Source: three-view drawing plus pictorial views. Frame: mm from the lowest corner of the part. Give positions to 0.01 mm unless a question says otherwise; leave off trailing zeros. Write each loop counter-clockwise with the first axis right and the second up, starting at its lowest first coordinate (ties: lowest second). Pieces come first, ordered by that corner, then holes.
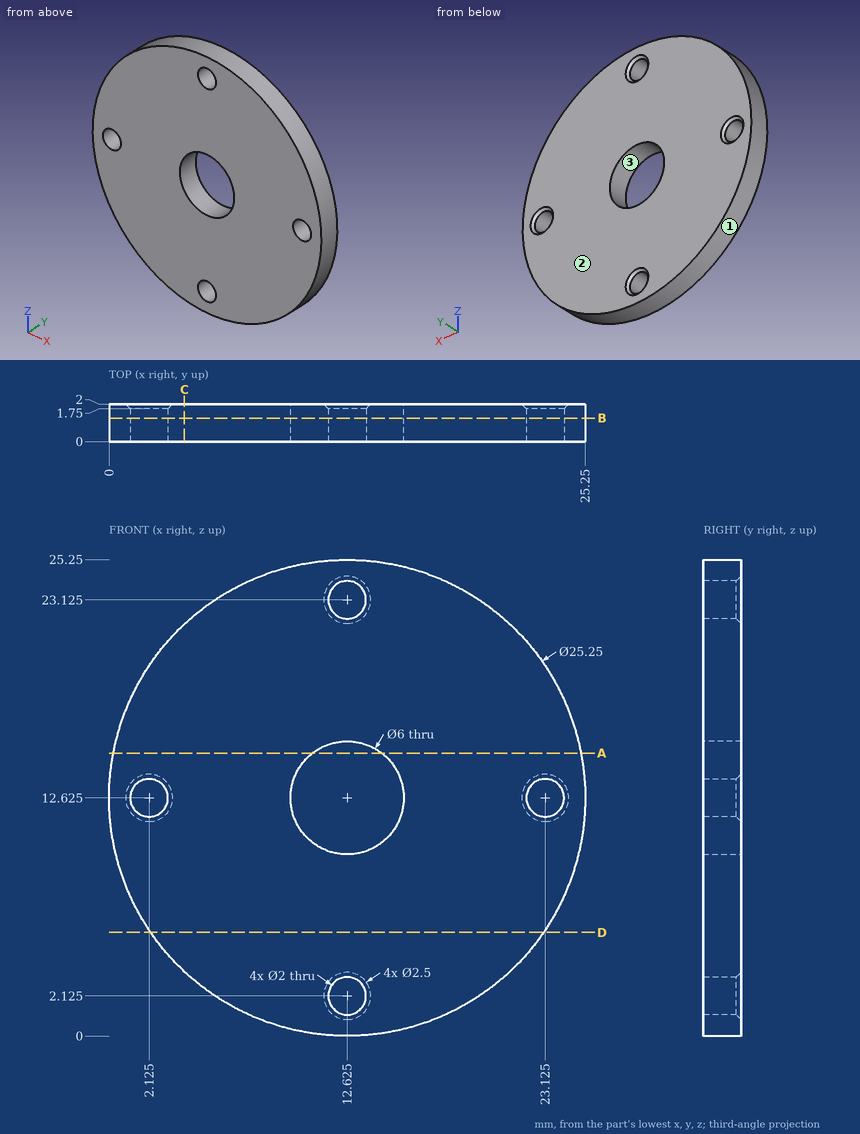
Q1. Section D-D on z = 5.5. Output: boundary loops of the cut face in (x, y), plus the area to 3 significant figures.
Filled sheet:
outline: (2.2, 0) - (23.05, 0) - (23.05, 2) - (2.2, 2) - close
area: 41.7 mm2
Q2. Ray query, line 1 along X through (y, z) = (1.75, 8); line 2 along X through (y, z) = (0.15, 13); line 3 along X through (y, z) = (0.5, 14.5). Return the intervals inside material, ascending.
Filled sheet:
line 1: x = 0.88 to 24.37
line 2: x = 0.01 to 1.2, 3.05 to 9.65, 15.6 to 22.2, 24.05 to 25.24
line 3: x = 0.14 to 10.28, 14.97 to 25.11
Q3. Section B-B on y = 1.25. Output: boundary loops of the cut face in (x, z) (3 decimals).
Filled sheet:
outline: circle Ø25.25 at (12.625, 12.625); hole circle Ø2 at (2.125, 12.625); hole circle Ø6 at (12.625, 12.625); hole circle Ø2 at (12.625, 2.125); hole circle Ø2 at (12.625, 23.125); hole circle Ø2 at (23.125, 12.625)
Q4. Pull-direction query (Z, two-part tool) for the marked faces 1, 2 and 3; classes: released by +Z, released by -Z, zero draft, split by the parting line, or undercut.
Filled sheet:
face 1: split by the parting line
face 2: zero draft
face 3: undercut
Q5. Section A-A on z = 15. Output: boundary loops of the cut face in (x, y), plus the area to 3 significant figures.
Filled sheet:
outline: (0.23, 0) - (10.79, 0) - (10.79, 2) - (0.23, 2) - close; (14.46, 0) - (25.02, 0) - (25.02, 2) - (14.46, 2) - close
area: 42.3 mm2
Q6. Section C-C on x = 4. Output: boundary loops of the cut face in (y, z).
Filled sheet:
outline: (0, 3.41) - (2, 3.41) - (2, 21.84) - (0, 21.84) - close
